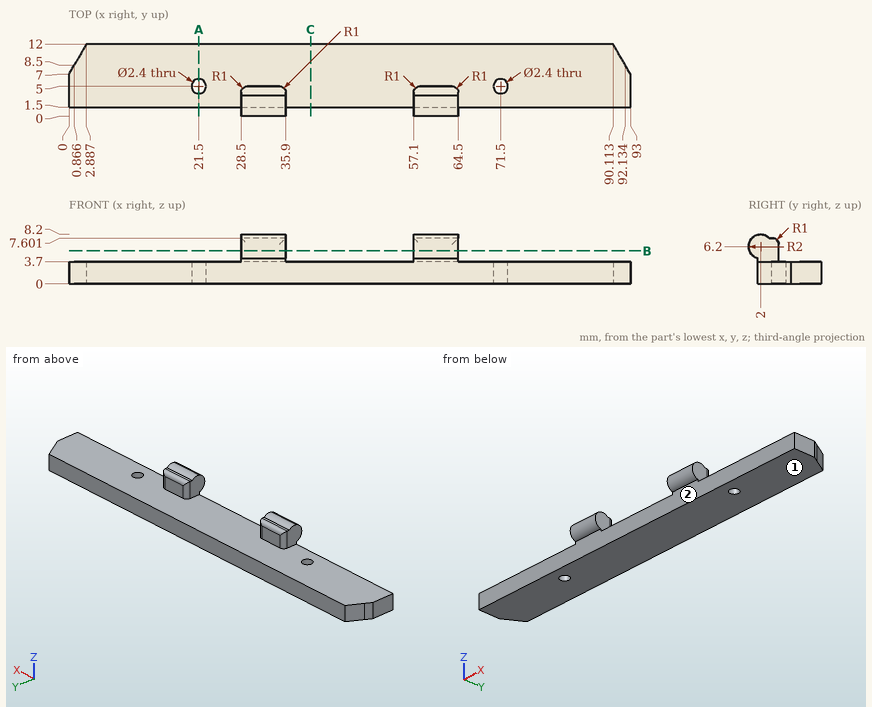
Geometry: see drawing. Coordinates: mm, zero at the bounding-box minimum. A direction names the side the tool comes from. Coordinates: 2 decimals unless noted, no trailing zeros. Order: outer loops, then holes, each group sorted by start corner. A loop starts at its lowest first (then second) coordinate and runs counter-clockwise, first axis right, second up. Notation, with made-up numbers: (39, 0.25) -> (43, 0.25) arc R5 ccw to (43, 5.25) -> close; hole circle Ø7 at (-0.75, 59). An arc over 180 degrees is marked (long way). Write each question's results on one line, items separated by ' | '. Start each with the question number.
1) Cut plane C-C, the plane x = 40. Output: boundary loops of the cut face in (y, z).
2) Cut plane B-B, the plane z = 5.5. Output: boundary loops of the cut face in (x, y).
3) First-contact query: pin 1 (0.6 mm diameter, centred on x = 61.5, y = 4, fed in from +Z); pin 2 (0.6 mm diameter, centred on x = 34, y = 3.5, fed in from +Z); pin 3 (3 mm diameter, centred on x = 30, z = 1.5, fed in from -Y). Flat tips, straight axial feed; report the tip coordinate or a pass-through.
4) Cut plane A-A, the plane x = 21.5. Output: boundary loops of the cut face in (y, z), and give its area (3 significant figures).
5) Material intervals for line 1 along Y through (x, z) = (71.5, 2.25); line 2 along X through (y, z) = (1.5, 6.25); line 3 along Z through (x, y) = (22.5, 2.75), sorted ascending.
6) Set-up query: the marked faces 1 and 2. Return all of +Z, -Z, +X, -X, +Y, -Y with unobstructed straight access to the full face (end or side cutting, diameter ignored); none if empty.
Checks:
1) outline: (1.5, 0) -> (12, 0) -> (12, 3.7) -> (1.5, 3.7) -> close
2) outline: (28.5, 0.13) -> (35.9, 0.13) -> (35.9, 4) arc R1 ccw to (34.9, 5) -> (29.5, 5) arc R1 ccw to (28.5, 4) -> close; (57.1, 0.13) -> (64.5, 0.13) -> (64.5, 4) arc R1 ccw to (63.5, 5) -> (58.1, 5) arc R1 ccw to (57.1, 4) -> close
3) pin 1: z = 7.6 | pin 2: z = 7.8 | pin 3: y = 1.5
4) outline: (1.5, 0) -> (3.8, 0) -> (3.8, 3.7) -> (1.5, 3.7) -> close; (6.2, 0) -> (12, 0) -> (12, 3.7) -> (6.2, 3.7) -> close | area: 30.0 mm^2
5) line 1: 1.5 to 3.8, 6.2 to 12 | line 2: 28.5 to 35.9, 57.1 to 64.5 | line 3: 0 to 3.7
6) face 1: -Z, +X, -X, +Y, -Y | face 2: -Z, +X, -X, -Y
